from build123d import *

# Parameters (mm, degrees)
SKETCH_1_R           = 2.9
SKETCH_1_R_2         = 1.1
EXTRUDE_1_DEPTH      = 3
SKETCH_2_R           = 4.5
CUT_EXTRUDE_1_DEPTH  = 1.5
SKETCH_3_W           = 49
SKETCH_3_H           = 4
EXTRUDE_2_DEPTH      = 24
EXTRUDE_2_DEPTH_BACK = 14
SKETCH_4_W           = 22
SKETCH_4_H           = 8
SKETCH_4_R           = 1.3
SKETCH_4_R_2         = 10
CUT_EXTRUDE_7_DEPTH  = 5
CUT_EXTRUDE_8_DEPTH  = 2


with BuildPart() as part:
    # 草图1 → 凸台-拉伸1 (new body)
    with BuildSketch(Plane(origin=(0, 0, 0), x_dir=(1, 0, 0), z_dir=(0, 1, 0))):
        Polygon((-42, 50.3), (-42, 3.3), (-42, -43.7), (0, -43.7), (7, -43.7), (7, 47), (7, 67), (-42, 67), align=None)
        with Locations((-35, -40)):
            Circle(SKETCH_1_R, mode=Mode.SUBTRACT)
        with Locations((-34, -30)):
            Circle(SKETCH_1_R_2, mode=Mode.SUBTRACT)
        Polygon((-35, -25), (-35, -4), (-21.05, -4), (-21.05, -40), (-25.5, -40), (-25.5, -25), align=None, mode=Mode.SUBTRACT)
        Polygon((-1.1, -4), (-1.1, -25), (-10.6, -25), (-10.6, -40), (-15.05, -40), (-15.05, -4), align=None, mode=Mode.SUBTRACT)
        with Locations((0, -40)):
            Circle(SKETCH_1_R, mode=Mode.SUBTRACT)
        with Locations((-1.1, -30)):
            Circle(SKETCH_1_R_2, mode=Mode.SUBTRACT)
        with Locations((-34, 30)):
            Circle(SKETCH_1_R_2, mode=Mode.SUBTRACT)
        Polygon((-21.05, 4), (-35, 4), (-35, 25.5), (-25.5, 25.5), (-25.5, 40), (-21.05, 40), align=None, mode=Mode.SUBTRACT)
        with Locations((-35, 40)):
            Circle(SKETCH_1_R, mode=Mode.SUBTRACT)
        Polygon((-10.6, 25.5), (-1.1, 25.5), (-1.1, 4), (-15.05, 4), (-15.05, 40), (-10.6, 40), align=None, mode=Mode.SUBTRACT)
        with Locations((-1.1, 30)):
            Circle(SKETCH_1_R_2, mode=Mode.SUBTRACT)
        with Locations((0, 40)):
            Circle(SKETCH_1_R, mode=Mode.SUBTRACT)
    extrude(amount=EXTRUDE_1_DEPTH)

    # 草图2 → 切除-拉伸1 (cut)
    with BuildSketch(Plane(origin=(0, 3, 0), x_dir=(1, 0, 0), z_dir=(0, 1, 0))):
        with Locations((-35, 40)):
            Circle(SKETCH_2_R)
        with Locations((0, 40)):
            Circle(SKETCH_2_R)
        with Locations((0, -40)):
            Circle(SKETCH_2_R)
        with Locations((-35, -40)):
            Circle(SKETCH_2_R)
    extrude(amount=-CUT_EXTRUDE_1_DEPTH, mode=Mode.SUBTRACT)

    # 草图3 → 凸台-拉伸2 (add, two sides)
    with BuildSketch(Plane(origin=(0, 3, 0), x_dir=(1, 0, 0), z_dir=(0, 1, 0))) as extrude_2_sk:
        with Locations((-17.5, 69)):
            Rectangle(SKETCH_3_W, SKETCH_3_H)
    extrude(amount=EXTRUDE_2_DEPTH)
    extrude(extrude_2_sk.sketch, amount=-EXTRUDE_2_DEPTH_BACK)

    # 草图4 → 切除-拉伸7 (cut, through all)
    with BuildSketch(Plane.XY.offset(-67)):
        with Locations((-17.95, -5.5)):
            Rectangle(SKETCH_4_W, SKETCH_4_H)
        with Locations((-31.75, 22)):
            Circle(SKETCH_4_R)
        with Locations((-3.25, 22)):
            Circle(SKETCH_4_R)
        with Locations((-2.75, -6.5)):
            Circle(SKETCH_4_R)
        with Locations((-32.25, -6.5)):
            Circle(SKETCH_4_R)
        with Locations((-17.5, 15)):
            Circle(SKETCH_4_R_2)
    extrude(amount=-CUT_EXTRUDE_7_DEPTH, mode=Mode.SUBTRACT)

    # 草图5 → 切除-拉伸8 (cut)
    with BuildSketch(Plane(origin=(0, 0, -71), x_dir=(-1, 0, 0), z_dir=(0, 0, -1))):
        Polygon((2.113595541, 22.631335811), (2.113595541, 23.270329273), (32.026158538, 23.270329273), (33.610999862, 23.270329273), (33.610999862, -7.824323718), (2.113595541, -7.824323718), align=None)
    extrude(amount=-CUT_EXTRUDE_8_DEPTH, mode=Mode.SUBTRACT)


solid = part.part
Work out the finished part from the listing and answer in its coordinate system (mm). A direction names the side the tool comes from. Round coordinates to 2 decimals unless told otherwise and drop trailing zeros. Write each loop counter-clockwise with the first axis right and the second up, starting at its lowest first coordinate (ties: lowest second). Pieces come first, ordered by that corner, then holes.
1) A tool of negligible diameter and unlimited length cuts with its end or side. For faces 4 (the flat face through (-1.1, 1, -15)), 5 (the flat face through (-18, -1, -67)), 6 (the flat face through (-18, 4, -67)), 7 (the flat face through (-27, 23.27, -70)), 8 (the flat face through (7, 2, -30)), from which of +Z, -Z, +X, -X, +Y, -Y can it reach the whole face along a straight path? Write none if from no direction.
2) A cutting plane is placed at C-C (x = -16.5). Give the vertices of the cut face in (y, z), plus the area to 3 significant figures.
3) A cutting plane is placed at A-A (z = 30). Give the vertices of the cut face in (x, y).
4) A cutting plane is placed at D-D (y = 8). Give the vertices of the cut face in (x, z).
5) The mould has two halves that part along Y. Classify faces 1 (the cylindrical face through (-33.55, -6.44, -67.99)), 2 (the flat face through (-32, 1.5, -39)), 3 (the flat face through (-1.1, 1, 14)): pulls with the +Y half, pulls with the -Y half, needs draft (parallel to the pull), parting line crosses it, or undercut.
6) Straight lines are drawn through the part: line 1 (X direction, y = 2, z = -30); line 2 (Z direction, x = -1, y = 1); line 3 (X direction, y = 2, z = -37). For each, find the intervals that lie inside material, in ascending order.
7) A cutting plane is placed at B-B (y = -6.5). Give the vertices of the cut face in (x, z).
8) Given pin 1 Ø5 at (x, z) = (-24.5, -28) entering from +Y; pin 2 Ø1.5 at (x, y) = (-8.5, 1) entering from -Z; pin 3 Ø1.5 at (x, y) = (-31, 7.5) entering from +Z, each flat-ended and moving along its own axis, determine where each tip first touches the part or whether it passes through.
Completed:
1. face 4: +Y, -Y
1. face 5: +Z, +X, -X, -Y
1. face 6: +Z, +X, -X, +Y
1. face 7: -Z
1. face 8: +Z, -Z, +X, +Y, -Y
2. outline: (-11, -71) - (-9.5, -71) - (-9.5, -67) - (-11, -67) - close; (-1.5, -69) - (5.05, -69) - (5.05, -67) - (3, -67) - (3, 43.7) - (0, 43.7) - (0, -67) - (-1.5, -67) - close; (24.95, -71) - (27, -71) - (27, -67) - (24.95, -67) - close
2. area: 359 mm2
3. outline: (-42, 0) - (-35.1, 0) - (-35.1, 3) - (-42, 3) - close; (-32.9, 0) - (-25.5, 0) - (-25.5, 3) - (-32.9, 3) - close; (-21.05, 0) - (-15.05, 0) - (-15.05, 3) - (-21.05, 3) - close; (-10.6, 0) - (-2.2, 0) - (-2.2, 3) - (-10.6, 3) - close; (0, 0) - (7, 0) - (7, 3) - (0, 3) - close
4. outline: (-42, -71) - (-33.61, -71) - (-33.61, -69) - (-24.64, -69) - (-24.64, -67) - (-42, -67) - close; (-10.36, -69) - (-2.11, -69) - (-2.11, -71) - (7, -71) - (7, -67) - (-10.36, -67) - close
5. face 1: undercut
5. face 2: pulls with the +Y half
5. face 3: needs draft
6. line 1: x = -42 to -35.1, -32.9 to -25.5, -21.05 to -15.05, -10.6 to -2.2, 0 to 7
6. line 2: z = -71 to -42.72, -37.28 to -31.1, -28.9 to 28.9, 31.1 to 37.28, 42.72 to 43.7
6. line 3: x = -42 to -38.35, -31.65 to -25.5, -21.05 to -15.05, -10.6 to -3.35, 3.35 to 7
7. outline: (-42, -71) - (-33.61, -71) - (-33.61, -69) - (-33.55, -69) - (-33.55, -67) - (-42, -67) - close; (-30.95, -69) - (-28.95, -69) - (-28.95, -67) - (-30.95, -67) - close; (-6.95, -69) - (-4.05, -69) - (-4.05, -67) - (-6.95, -67) - close; (-1.45, -71) - (7, -71) - (7, -67) - (-1.45, -67) - close
8. pin 1: stops at y = 3
8. pin 2: stops at z = -69
8. pin 3: stops at z = -67
